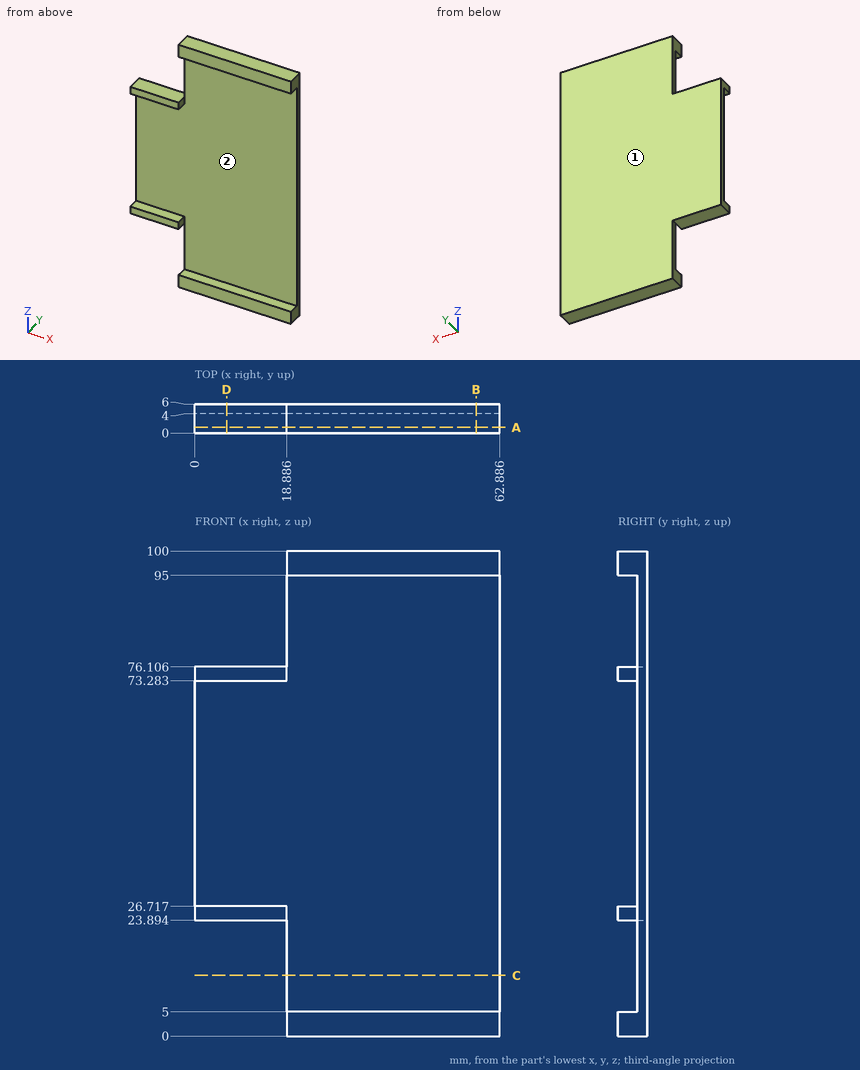
Verification items for this drawing (mm, ordinates from the low corner). Give positions to 0.01 mm unless a question says otherwise; leave off trailing zeros. Write each loop counter-clockwise with the first axis right and the second up, starting at its lowest first coordinate (ties: lowest second). Pieces come first, ordered by that corner, then holes.
1) Cross-section at C-C (z = 12.5). Record the boundary of the cut face in (x, y).
Values follow:
outline: (18.89, 4) - (62.89, 4) - (62.89, 6) - (18.89, 6) - close
2) Go/stop test with flat-tipped pins: pin 1 Ø3 at (x, z) = (40, 74.5) entering from -Y; pin 2 Ø3 at (x, y) = (11.5, 2) entering from +Z; pin 3 Ø1.5 at (y, z) = (2, 60.5) entering from -X; pin 4 Ø2 at (x, y) = (11, 3) entering from -Z. Record where each tip stops, or that it passes through.
Values follow:
pin 1: stops at y = 4
pin 2: stops at z = 76.11
pin 3: passes through
pin 4: stops at z = 23.89
3) Cross-section at D-D (x = 6.5). Record the boundary of the cut face in (y, z).
Values follow:
outline: (0, 23.89) - (6, 23.89) - (6, 76.11) - (0, 76.11) - (0, 73.28) - (4, 73.28) - (4, 26.72) - (0, 26.72) - close
4) Release check for a two-part mould opening along Z. For the marked faces 1 and 2 record: released by +Z, released by -Z, zero draft, split by the parting line, or undercut.
Values follow:
face 1: zero draft
face 2: undercut
5) Cross-section at B-B (x = 58). Record the boundary of the cut face in (y, z), plus the area to 3 significant figures.
Values follow:
outline: (0, 0) - (6, 0) - (6, 100) - (0, 100) - (0, 95) - (4, 95) - (4, 5) - (0, 5) - close
area: 240 mm2
6) Thickness scan on line 1 (Z direction, x = 52, y = 3.25); line 2 (Z direction, x = 14, y = 3.05); line 3 (Y direction, x = 30, z = 16.5). Record the ranges inside material, lowest first.
Values follow:
line 1: z = 0 to 5, 95 to 100
line 2: z = 23.89 to 26.72, 73.28 to 76.11
line 3: y = 4 to 6
7) Cross-section at A-A (y = 1.2). Record the boundary of the cut face in (x, z).
Values follow:
outline: (0, 23.89) - (18.89, 23.89) - (18.89, 26.72) - (0, 26.72) - close; (0, 73.28) - (18.89, 73.28) - (18.89, 76.11) - (0, 76.11) - close; (18.89, 0) - (62.89, 0) - (62.89, 5) - (18.89, 5) - close; (18.89, 95) - (62.89, 95) - (62.89, 100) - (18.89, 100) - close
